Could you check a few things on this model? Use its own coordinates, in mm. Face numbers are marked on the shaded views. A direction names the side the tool comes from. Coordinates: 2 decimals unless noted, no trailing zeros. Loops run counter-clockwise (first coordinate to the right, second up) from the corner with the lowest first, then second, coordinate; pieces in that order, holes last. Notation, with made-up numbers: (38.5, 8.25) - (43.5, 8.25) arc R34 ccw to (43.5, 38.25) - close; hole circle Ø11 at (38.5, 17.25). An arc over 180 degrees is marked (long way). One line per item, written item: value. Start each with the question number.
(1) If we section it at A-A on y = -23.5: Write out the boundary of the cut face in (x, z), then the cut area to 3 significant figures.
(2) If I drill on line 1 along Y through (x, z) = (-35, -2); line 2 along X through (y, z) = (-21.5, 7); line 3 along Z through (x, y) = (-11.5, -10.5), over which ranges is the centre line in solid material (lowest first)? Write a range as from..to.
(3) If we mould it in two halves opening along X, with no side actions, what happens to the marked faces 4, 5 and 6? For each: pulls with the +X half, pulls with the -X half, needs draft (parallel to the pull), parting line crosses it, or undercut.
(4) If we section it at D-D on y = -16: Write out the boundary of the cut face in (x, z), then the cut area to 3 significant figures.
(5) If we section it at C-C on z = 11.5: Write out the boundary of the cut face in (x, y), then the cut area to 3 significant figures.
(6) If we section it at B-B on x = 35.25: Write out the boundary of the cut face in (y, z), then the cut area to 3 significant figures.
(7) On a 3-axis mill with a long thin cutter (end or side, diameter ignored), from which of +Z, -Z, +X, -X, +Y, -Y can I reach the whole of each face in a straight line? I mean the marked faces 1, 2 and 3. Say none if no direction works.
(8) I'm going to push flat-ended pins straight in: P1, Ø1, axis at x = 6.5, y = -6, coming from the -Z side; P2, Ø2.5, axis at x = -33.5, y = -16, coming from the +Z side; P3, Ø10, axis at y = -18, z = 17, coming from the -X side. Where does each tip first touch, or does it pass through?
```python
from build123d import *

# Parameters (mm, degrees)
F1_DEPTH = 30
F2_R     = 2.2479
F3_DEPTH = 3.5
F4_R     = 1.5


# Not quite as in the source:
# - a pattern or mirror of a feature is missing from the dataset's text; its kind, count and spacing are read off the source's solid


with BuildPart() as f1:
    # F0 (on Front) → F1 (new body)
    with BuildSketch(Plane.XZ):
        Polygon((-26, 0), (-26, 31.5), (26, 31.5), (26, 0), (29.5, 0), (29.5, 35), (-29.5, 35), (-29.5, 0), align=None)
        Polygon((-26, -3.5), (-26, 0), (-29.5, 0), (-41, 0), (-41, -3.5), align=None)
        Polygon((29.5, 0), (26, 0), (26, -3.5), (41, -3.5), (41, 0), align=None)
    extrude(amount=F1_DEPTH)

    # F2 (on face) → F3 (cut, through all)
    with BuildSketch(Plane.XY):
        with Locations((-35.25, -23.5)):
            Circle(F2_R)
        with Locations((-35.25, -6.5)):
            Circle(F2_R)
    f3 = extrude(amount=-F3_DEPTH, mode=Mode.SUBTRACT)

    # F3_copies: F3 across plane
    add(f3.mirror(Plane(origin=(0, 0, 0), x_dir=(0, 0, 1), z_dir=(1, 0, 0))), mode=Mode.SUBTRACT)

    # F4
    f4_edges = [f1.edges().sort_by_distance(p)[0] for p in [
        (-29.5, -15, 35),
        (-29.5, -15, 0),
        (-41, -15, 0),
        (29.5, -15, 35),
        (29.5, -15, 0),
        (41, -15, 0),
    ]]
    fillet(f4_edges, radius=F4_R)


solid = f1.part
```
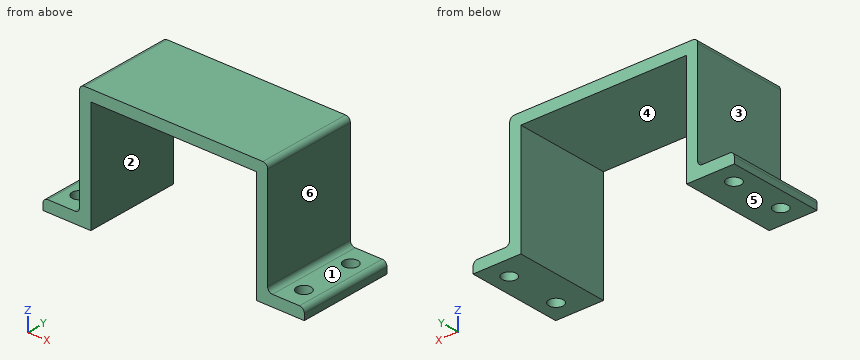
Values:
1. outline: (-41, -3.5) - (-37.5, -3.5) - (-37.5, 0) - (-39.5, 0) arc R1.5 ccw to (-41, -1.5) - close; (-33, -3.5) - (-26, -3.5) - (-26, 31.5) - (26, 31.5) - (26, -3.5) - (33, -3.5) - (33, 0) - (31, 0) arc R1.5 cw to (29.5, 1.5) - (29.5, 33.5) arc R1.5 ccw to (28, 35) - (-28, 35) arc R1.5 ccw to (-29.5, 33.5) - (-29.5, 1.5) arc R1.5 cw to (-31, 0) - (-33, 0) - close; (37.5, -3.5) - (41, -3.5) - (41, -1.5) arc R1.5 ccw to (39.5, 0) - (37.5, 0) - close
1. area: 500 mm2
2. line 1: y = -30..-25.73, -21.27..-8.73, -4.27..0
2. line 2: x = -29.5..-26, 26..29.5
2. line 3: z = 31.5..35
3. face 4: undercut
3. face 5: needs draft
3. face 6: pulls with the +X half
4. outline: (-41, -3.5) - (-26, -3.5) - (-26, 31.5) - (26, 31.5) - (26, -3.5) - (41, -3.5) - (41, -1.5) arc R1.5 ccw to (39.5, 0) - (31, 0) arc R1.5 cw to (29.5, 1.5) - (29.5, 33.5) arc R1.5 ccw to (28, 35) - (-28, 35) arc R1.5 ccw to (-29.5, 33.5) - (-29.5, 1.5) arc R1.5 cw to (-31, 0) - (-39.5, 0) arc R1.5 ccw to (-41, -1.5) - close
4. area: 531 mm2
5. outline: (-29.5, -30) - (-26, -30) - (-26, 0) - (-29.5, 0) - close; (26, -30) - (29.5, -30) - (29.5, 0) - (26, 0) - close
5. area: 210 mm2
6. outline: (-30, -3.5) - (-25.75, -3.5) - (-25.75, 0) - (-30, 0) - close; (-21.25, -3.5) - (-8.75, -3.5) - (-8.75, 0) - (-21.25, 0) - close; (-4.25, -3.5) - (0, -3.5) - (0, 0) - (-4.25, 0) - close
6. area: 73.5 mm2
7. face 1: +Z, +X, +Y, -Y
7. face 2: -Z, +Y, -Y
7. face 3: +Z, -X, +Y, -Y
8. P1: stops at z = 31.5
8. P2: stops at z = 0
8. P3: stops at x = -29.5
